The listing builds one solid part. Answer for the finished solid, in the listing's coordinates (mm). A direction names the side the tool comes from. Coordinates: 2 decimals unless noted, no trailing zeros. Write each loop counter-clockwise with the first axis right and the second up, starting at its lowest first coordinate (ties: lowest second). Pieces come first, ordered by that corner, then holes.
(1) Which of the six approach directions +Z, -Z, +X, -X, +Y, -Y give full straight-line access (tool end or side, diameter ignored) to faces 1 (the flat face through (0, 3, -8.382)), 2 (the cylindrical face through (0.046, 2.504, -5.627))?
(2) For a pull along Z with two mould halves and no side action, classify faces 3 (the flat face through (2.569, 3, 0)), 4 (the flat face through (0, 3, 8.382)), 5 (the flat face through (19.05, 3, 0)) as +Z half, -Z half, draft (parallel to the pull), parting line (faces both ways), or undercut.
(3) Straight lines are drawn through the part: line 1 (X direction, y = 3, z = 0); line 2 (Z direction, x = 15, y = 0.5); line 3 (X direction, y = 2.1, z = 2.25). For each, find the intervals that lie inside material, in ascending order.
(4) The part is cut by section B-B on y = 2.2. Determine the outline of the cut face in (x, z), plus the area to 3 significant figures.
(5) The part is cut by section C-C on z = 0. Determine the outline of the cut face in (x, y), plus the area to 3 significant figures.
(6) Given P1, Ø2, axis at x = -10.01, z = 0, coming from the +Y side, flat-ended and moving along its own axis, determine where the tip first touches the part or whether it passes through.
(7) The part is cut by section A-A on z = -2.5. Determine the outline of the cut face in (x, y), plus the area to 3 significant figures.
(8) The part is cut by section D-D on x = -9.5. Determine the outline of the cut face in (y, z).
from build123d import *

# Parameters (mm, degrees)
SKETCH1_W           = 38.1
SKETCH1_H           = 16.764
SKETCH1_R           = 1.2446
BOSS_EXTRUDE1_DEPTH = 5.08


with BuildPart() as part:
    # Sketch1 → Boss-Extrude1 (new body)
    with BuildSketch(Plane(origin=(0, 0, 0), x_dir=(1, 0, 0), z_dir=(0, 1, 0))):
        Rectangle(SKETCH1_W, SKETCH1_H)
        with Locations((-10.0076, 0)):
            Circle(SKETCH1_R, mode=Mode.SUBTRACT)
        with Locations((-15.0114, 0)):
            Circle(SKETCH1_R, mode=Mode.SUBTRACT)
        with Locations((15.0114, 0)):
            Circle(SKETCH1_R, mode=Mode.SUBTRACT)
        with Locations((10.0076, 0)):
            Circle(SKETCH1_R, mode=Mode.SUBTRACT)
        with BuildLine():
            Line((2.568575, -3.048), (2.568575, 3.048))
            ThreePointArc((2.568575, 3.048), (-0.0111125, 5.6276875), (-2.5908, 3.048))
            Line((-2.5908, 3.048), (-2.5908, -3.048))
            ThreePointArc((-2.5908, -3.048), (-0.0111125, -5.6276875), (2.568575, -3.048))
        make_face(mode=Mode.SUBTRACT)
    extrude(amount=BOSS_EXTRUDE1_DEPTH)


solid = part.part
Model answer:
1. face 1: -Z, +X, -X, +Y, -Y
1. face 2: +Y, -Y
2. face 3: undercut
2. face 4: +Z half
2. face 5: draft
3. line 1: x = -19.05 to -16.26, -13.77 to -11.25, -8.76 to -2.59, 2.57 to 8.76, 11.25 to 13.77, 16.26 to 19.05
3. line 2: z = -8.38 to -1.24, 1.24 to 8.38
3. line 3: x = -19.05 to -2.59, 2.57 to 19.05
4. outline: (-19.05, -8.38) - (19.05, -8.38) - (19.05, 8.38) - (-19.05, 8.38) - close; hole circle Ø2.49 at (-15.01, 0); hole circle Ø2.49 at (-10.01, 0); hole (-2.59, -3.05) arc R2.58 ccw to (2.57, -3.05) - (2.57, 3.05) arc R2.58 ccw to (-2.59, 3.05) - close; hole circle Ø2.49 at (10.01, 0); hole circle Ø2.49 at (15.01, 0)
4. area: 567 mm2
5. outline: (-19.05, 0) - (-16.26, 0) - (-16.26, 5.08) - (-19.05, 5.08) - close; (-13.77, 0) - (-11.25, 0) - (-11.25, 5.08) - (-13.77, 5.08) - close; (-8.76, 0) - (-2.59, 0) - (-2.59, 5.08) - (-8.76, 5.08) - close; (2.57, 0) - (8.76, 0) - (8.76, 5.08) - (2.57, 5.08) - close; (11.25, 0) - (13.77, 0) - (13.77, 5.08) - (11.25, 5.08) - close; (16.26, 0) - (19.05, 0) - (19.05, 5.08) - (16.26, 5.08) - close
5. area: 117 mm2
6. P1: passes through
7. outline: (-19.05, 0) - (-2.59, 0) - (-2.59, 5.08) - (-19.05, 5.08) - close; (2.57, 0) - (19.05, 0) - (19.05, 5.08) - (2.57, 5.08) - close
7. area: 167 mm2
8. outline: (0, -8.38) - (5.08, -8.38) - (5.08, -1.14) - (0, -1.14) - close; (0, 1.14) - (5.08, 1.14) - (5.08, 8.38) - (0, 8.38) - close
